The listing builds one solid part. Answer for the finished solid, in the listing's coordinates (mm). Face numbers are marked on the shaded views. A direction names the side the tool comes from. Give positions to 0.01 mm unless a question says otherwise; leave off trailing zeros. Write each loop counter-clockwise with the first axis right and the second up, starting at its lowest first coordinate (ties: lowest second). Pieces come first, ordered by that corner, then holes. Notation, with made-up numbers: (20, 15) - (31, 15) arc R24 cw to (31, 41) - close; hole circle Ø8 at (83, 67.25). An arc over 180 degrees is marked (long way). Return JSON: item names as keys, results as strings.
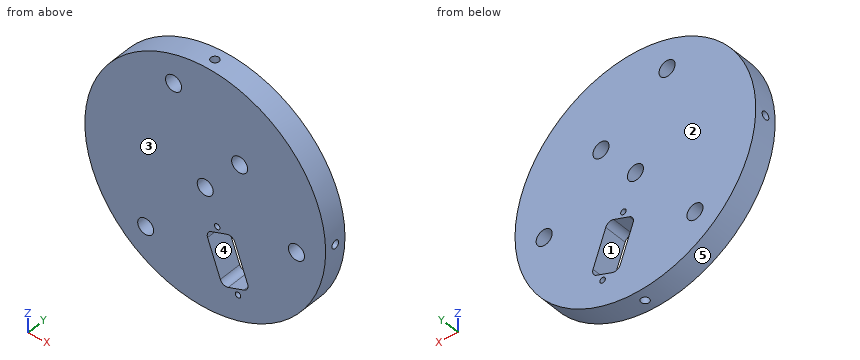
from build123d import *

# Parameters (mm, degrees)
SKETCH1_R                 = 78.359
SKETCH1_R_2               = 51.1048
BOSS_EXTRUDE1_DEPTH       = 25.4
SKETCH6_R                 = 49.5173
BOSS_EXTRUDE5_DEPTH       = 9.525
SKETCH7_R                 = 49.5173
BOSS_EXTRUDE6_DEPTH       = 9.525
SKETCH9_R                 = 3.3
CUT_EXTRUDE6_DEPTH        = 45.45
SKETCH10_R                = 82.322787435
CUT_EXTRUDE7_DEPTH        = 35.925
TAP_DRILL_FOR_4_40_TAP1_D = 2.2606
CUT_EXTRUDE9_DEPTH        = 10.525
CIRPATTERN1_COUNT         = 4


with BuildPart() as part:
    # Sketch1 → Boss-Extrude1 (new body)
    with BuildSketch(Plane(origin=(0, 0, 0), x_dir=(1, 0, 0), z_dir=(0, 1, 0))):
        Circle(SKETCH1_R)
        Circle(SKETCH1_R_2, mode=Mode.SUBTRACT)
    extrude(amount=BOSS_EXTRUDE1_DEPTH)


with BuildPart() as body_2:
    # Sketch6 → Boss-Extrude5 (new body)
    with BuildSketch(Plane(origin=(0, 25.4, 0), x_dir=(1, 0, 0), z_dir=(0, 1, 0))):
        Circle(SKETCH6_R)
    extrude(amount=BOSS_EXTRUDE5_DEPTH)


with BuildPart() as body_3:
    # Sketch7 → Boss-Extrude6 (new body)
    with BuildSketch(Plane.XZ):
        Circle(SKETCH7_R)
    extrude(amount=BOSS_EXTRUDE6_DEPTH)


with BuildPart() as cut_extrude6_tool:
    # Sketch9 → Cut-Extrude6 (new body, through all)
    with BuildSketch(Plane(origin=(0, 34.925, 0), x_dir=(1, 0, 0), z_dir=(0, 1, 0))):
        Circle(SKETCH9_R)
        with Locations((-13.030967461, -35.802288852)):
            Circle(SKETCH9_R)
        with Locations((14.149897915, -16.863191675)):
            Circle(SKETCH9_R)
        with Locations((-24.490207929, 29.186293283)):
            Circle(SKETCH9_R)
        with Locations((37.52117539, 6.615995569)):
            Circle(SKETCH9_R)
    extrude(amount=-CUT_EXTRUDE6_DEPTH)


with BuildPart() as body_2_1:
    add(body_2.part)

    # Cut-Extrude6: cut by cut_extrude6_tool
    add(cut_extrude6_tool.part, mode=Mode.SUBTRACT)

    # Tap Drill for #4-40 Tap1 (through all)
    with Locations(Plane(origin=(0, 34.925, 0), x_dir=(1, 0, 0), z_dir=(0, 1, 0))):
        with Locations((4.92280993, 13.525309122), (13.473313526, 37.017624677)):
            Hole(TAP_DRILL_FOR_4_40_TAP1_D / 2)

    # Sketch14 → Cut-Extrude9 (cut, through all)
    with BuildSketch(Plane(origin=(0, 34.925, 0), x_dir=(1, 0, 0), z_dir=(0, 1, 0))):
        with BuildLine():
            Line((12.182424395, 16.018747474), (17.431749568, 30.441149854))
            ThreePointArc((17.431749568, 30.441149854), (17.34695209, 32.383331403), (15.913661475, 33.696700275))
            Line((15.913661475, 33.696700275), (9.469249481, 36.042274418))
            ThreePointArc((9.469249481, 36.042274418), (7.527067933, 35.95747694), (6.213699061, 34.524186325))
            Line((6.213699061, 34.524186325), (0.964373888, 20.101783945))
            ThreePointArc((0.964373888, 20.101783945), (1.049171366, 18.159602396), (2.482461981, 16.846233524))
            Line((2.482461981, 16.846233524), (8.926873974, 14.500659381))
            ThreePointArc((8.926873974, 14.500659381), (10.869055523, 14.585456859), (12.182424395, 16.018747474))
        make_face()
    extrude(amount=-CUT_EXTRUDE9_DEPTH, mode=Mode.SUBTRACT)

    # Sketch17 → Tap Drill for M4x0.7 Tap1 (revolve, cut)
    with BuildSketch(Plane(origin=(49.5173, 30.1625, 0), x_dir=(0, 0, -1), z_dir=(0, 1, 0))):
        Polygon((0, 0), (0, 10.643420021), (1.65, 9.652), (1.65, 0), align=None)
    tap_drill_for_m4x0_7_tap1 = revolve(axis=Axis((55.8673, 30.1625, 0), (-1, 0, 0)), mode=Mode.SUBTRACT)

    # CirPattern1: Tap Drill for M4x0.7 Tap1 ×4 about axis
    cirpattern1_axis = Axis((0, 34.925, 0), (0, 1, 0))
    for i in range(1, CIRPATTERN1_COUNT):
        add(tap_drill_for_m4x0_7_tap1.rotate(cirpattern1_axis, i * 360 / CIRPATTERN1_COUNT), mode=Mode.SUBTRACT)


with BuildPart() as body_3_1:
    add(body_3.part)

    # Cut-Extrude6: cut by cut_extrude6_tool
    add(cut_extrude6_tool.part, mode=Mode.SUBTRACT)


with BuildPart() as cut_extrude7_tool:
    # Sketch10 → Cut-Extrude7 (new body, through all)
    with BuildSketch(Plane(origin=(0, 25.4, 0), x_dir=(1, 0, 0), z_dir=(0, 1, 0))):
        Circle(SKETCH10_R)
    extrude(amount=-CUT_EXTRUDE7_DEPTH)


with BuildPart() as part_1:
    add(part.part)

    # Cut-Extrude7: cut by cut_extrude7_tool
    add(cut_extrude7_tool.part, mode=Mode.SUBTRACT)


with BuildPart() as body_3_2:
    add(body_3_1.part)

    # Cut-Extrude7: cut by cut_extrude7_tool
    add(cut_extrude7_tool.part, mode=Mode.SUBTRACT)


solid = body_2_1.part
Item 1: Consider L1, parallel to Z at x = -42, y = 29.5; L2, parallel to Z at x = 39, y = 28.75; L3, parallel to X at y = 29.75, z = -23.5. Determine where each line is inside the solid, lowest interval first.
Answer below:
{"L1": "z = -26.23 to -1.51, 1.51 to 26.23", "L2": "z = -30.51 to -9.57, -3.67 to 30.51", "L3": "x = -43.59 to 2.2, 14.91 to 43.59"}
Item 2: A cutting plane is placed at C-C on x = 20.5. Determine the outline of the cut face in (y, z) (3 decimals).
Answer below:
{"outline": "(25.4, -45.075) - (34.925, -45.075) - (34.925, 45.075) - (25.4, 45.075) - close"}
Item 3: A cutting plane is placed at A-A on z = -23.5. Determine the outline of the cut face in (x, y) (3 decimals).
Answer below:
{"outline": "(-43.586, 25.4) - (2.201, 25.4) - (2.201, 34.925) - (-43.586, 34.925) - close; (14.905, 25.4) - (43.586, 25.4) - (43.586, 34.925) - (14.905, 34.925) - close"}
Item 4: For the marked faces 1 and 2, determine the directions among +Z, -Z, +X, -X, +Y, -Y from which every point of the face is accessible in a straight line to the end or side of a thin tool.
Answer below:
{"face 1": "+Y, -Y", "face 2": "+Z, -Z, +X, -X, +Y"}
Item 5: Flat-ended cylindrical pins translate along their axes: P1, Ø4.5, axis at y = 30.16, z = 0, coming from the -X side; P2, Ø3, axis at x = 0, y = 30.16, coming from the -Z side; P3, Ø5, axis at y = 30, z = 9, coming from the -X side; P4, Ø1.5, axis at y = 33, z = -39.5, coming from the -X side. Find the tip coordinate at first contact, or state that the pin passes through.
Answer below:
{"P1": "stops at x = -49.52", "P2": "stops at z = -39.78", "P3": "stops at x = -49.09", "P4": "stops at x = -30.83"}
Item 6: A cutting plane is placed at D-D on z = 30. Determine the outline of the cut face in (x, y) (3 decimals).
Answer below:
{"outline": "(-39.395, 25.4) - (39.395, 25.4) - (39.395, 34.925) - (-39.395, 34.925) - close"}
Item 7: The mould has two halves that part along X. Classify the marked faces 3, 4 and 5: +X half, -X half, draft (parallel to the pull), parting line (faces both ways), or undercut.
Answer below:
{"face 3": "draft", "face 4": "undercut", "face 5": "parting line"}
Item 8: A cutting plane is placed at B-B on z = 15.5. Determine the outline of the cut face in (x, y) (3 decimals).
Answer below:
{"outline": "(-47.029, 25.4) - (11.145, 25.4) - (11.145, 34.925) - (-47.029, 34.925) - close; (17.155, 25.4) - (47.029, 25.4) - (47.029, 34.925) - (17.155, 34.925) - close"}
